Read the model definition and answer for the solid it produces. Units are mm, in the model's axes. Face numbers are marked on the shaded views. A direction names the side the tool comes from. Coordinates: 2 decimals unless noted, no trailing zeros. Loops run counter-clockwise (first coordinate to the right, second up) from the corner with the lowest first, then second, coordinate; pieces in that order, holes last. Notation, with made-up numbers: M 50,-9 L 97,-9 A28 ccw 97,27 Z; hole C 17.25,-40 d6. An arc over 180 degrees is marked long. One line per item, written item: value. Start each with the question number.
Autodesk Inventor part; units mm, degrees
ref_plane "YZ Plane" through (0, 0, 0) normal (1, 0, 0) x (0, 1, 0)
ref_plane "XZ Plane" through (0, 0, 0) normal (0, 1, 0) x (-1, 0, 0)
ref_plane "XY Plane" through (0, 0, 0) normal (0, 0, 1) x (1, 0, 0)
sketch "Sketch1" plane through (0, 0, 0) normal (0, 0, 1) x (1, 0, 0)
  arc A0 (0, -5.25) -> (0, 5.25) centre (0, 0) ccw
  arc A1 (8.0777, 5) -> (0, 9.5) centre (0, 0) ccw
  line L0 (0, 0) -> (27.5, 0) construction
  arc A2 (27.5, 5) -> (27.5, -5) centre (27.5, 0) ccw construction
  line L1 (0, 9.5) -> (0, 5.25)
  line L2 (27.5, 5) -> (8.0777, 5)
  line L3 (27.5, -5) -> (8.0777, -5)
  arc A3 (27.5, -5) -> (27.5, 5) centre (27.5, 0) ccw
  circle A4 centre (27.5, 0) radius 2.25
  arc A5 (0, 9.5) -> (0, -9.5) centre (0, 0) ccw construction
  arc A6 (0, -9.5) -> (8.0777, -5) centre (0, 0) ccw
  arc A7 (0, 5.25) -> (0, -5.25) centre (0, 0) ccw construction
  line L4 (0, 5.25) -> (0, -5.25) construction
  line L5 (0, -5.25) -> (0, -9.5)
  dimension "d2" = 10
  dimension "d4" = 4.5
  dimension "d5" = 5.25
  dimension "d6" = 9.5
  dimension "d7" = 27.5
extrude "Extrusion1" add sketch "Sketch1" along normal mid plane 4
properties part number "garfo-1"
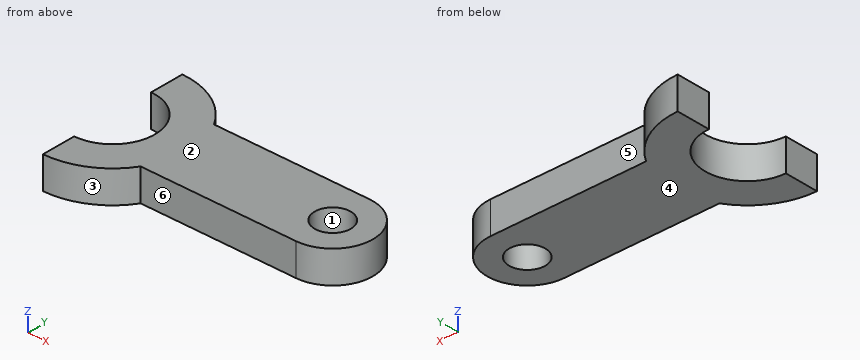
1) Section D-D (x = 17.5) is taken. Determine the outline of the cut face in (y, z).
2) Section B-B (z = 0.95) is taken. Determine the outline of the cut face in (x, y).
3) Section A-A (y = 0) is taken. Determine the outline of the cut face in (x, z), then the cut area to 3 significant figures.
4) For a pull along X with two mould halves and no side action, classify the marked faces 1, 2 and 3 as released by +X, released by -X, zero draft, split by the parting line, or undercut.
5) Consider line 1 along Y through (x, z) = (27.5, -0.05); line 2 along Y through (x, z) = (22.5, -1.2); line 3 along X through (y, z) = (-1.5, -1). Determine where each line is inside the solid, lowest interval first.
6) Section C-C (x = 26.5) is taken. Determine the outline of the cut face in (y, z), then the cut area to 3 significant figures.
7) A tool of negligible diameter and unlimited length cuts with its end or side. For the marked faces 4, 5 and 6, from which of +Z, -Z, +X, -X, +Y, -Y can it reach the whole face along a straight path? Write none if from no direction.
Results found:
1. outline: M -5,-2 L 5,-2 L 5,2 L -5,2 Z
2. outline: M 0,-9.5 A9.5 ccw 8.08,-5 L 27.5,-5 A5 ccw 27.5,5 L 8.08,5 A9.5 ccw 0,9.5 L 0,5.25 A5.25 cw 0,-5.25 Z; hole C 27.5,0 d4.5
3. outline: M 5.25,-2 L 25.25,-2 L 25.25,2 L 5.25,2 Z; M 29.75,-2 L 32.5,-2 L 32.5,2 L 29.75,2 Z
3. area: 91.0 mm²
4. face 1: undercut
4. face 2: zero draft
4. face 3: released by +X
5. line 1: y = -5 to -2.25, 2.25 to 5
5. line 2: y = -5 to 5
5. line 3: x = 5.03 to 25.82, 29.18 to 32.27
6. outline: M -5,-2 L -2.02,-2 L -2.02,2 L -5,2 Z; M 2.02,-2 L 5,-2 L 5,2 L 2.02,2 Z
6. area: 23.9 mm²
7. face 4: -Z, +X, -X, +Y, -Y
7. face 5: +Z, -Z, +X, +Y
7. face 6: +Z, -Z, +X, -Y
